Job drawing, mm, ordinate dimensions from the low corner. One solid piece. A direction names the side the tool comes from. Round coordinates to 2 decimals unless told otherwise and drop trailing zeros. Loops run counter-clockwise (first coordinate to the right, second up) from the corner with the lowest first, then second, coordinate; pieces in that order, holes last. Notation, with made-up numbers: M -8.75,57.5 L 6.25,57.5 A19 ccw 6.25,61.5 Z; hole C 40.25,71 d8. An arc over 180 degrees is marked long. One line per item, written item: value.
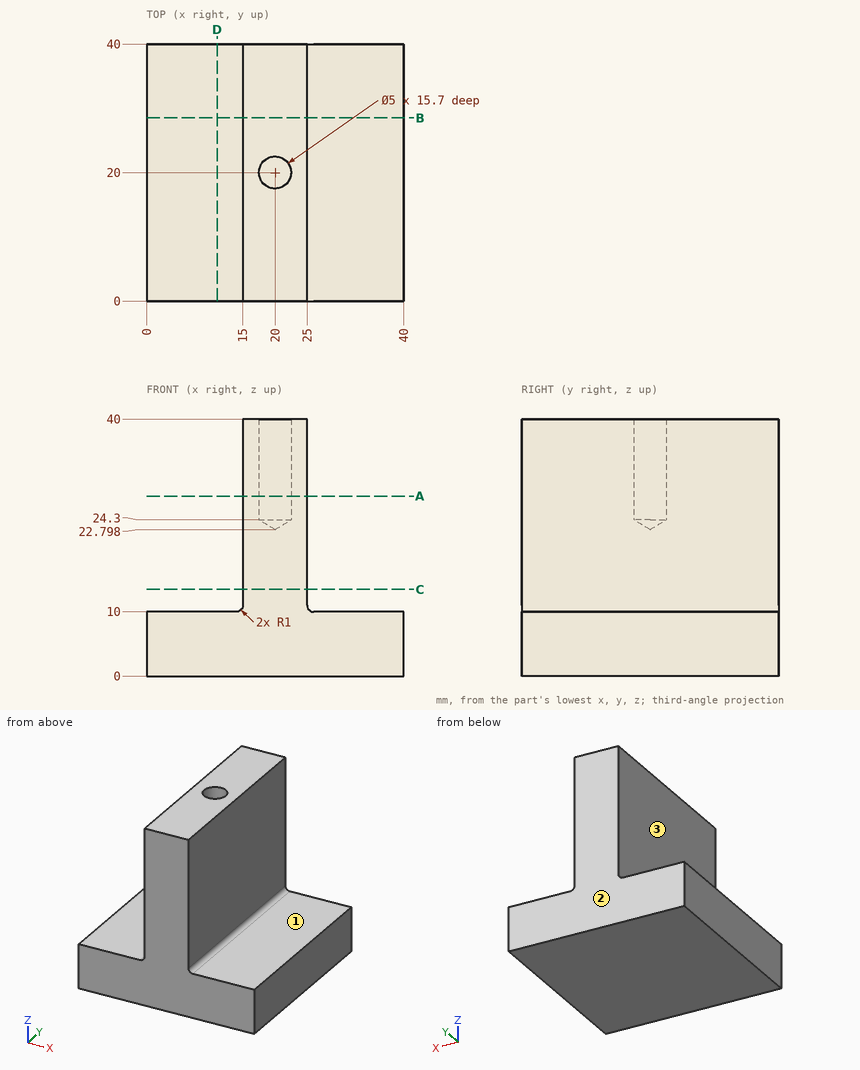
Item 1: Drop flat-ended pins along their axis: P1, Ø7, axis at x = 10, y = 11, coming from the +Z side; P2, Ø1.5, axis at y = 34, z = 12.5, coming from the +X side; P3, Ø14.5, axis at y = 25.5, z = 24, coming from the -X side. Give the stop position or say it passes through.
Check values:
P1: stops at z = 10
P2: stops at x = 25
P3: stops at x = 15
Item 2: Slice it at B-B, the plane y = 28.5. Give the cut face in (x, z).
Check values:
outline: M 0,0 L 40,0 L 40,10 L 26,10 A1 cw 25,11 L 25,40 L 15,40 L 15,11 A1 cw 14,10 L 0,10 Z
Item 3: Which spindle directions (+Z, -Z, +X, -X, +Y, -Y) get a long thin tool onto all of the face, cutting with end or side? Do the marked faces 1, 2 and 3. Say none if no direction does.
Check values:
face 1: +Z, +X, +Y, -Y
face 2: +Z, -Z, +X, -X, +Y
face 3: +Z, -X, +Y, -Y
Item 4: Slice it at C-C, the plane z = 13.5. Give the cut face in (x, y).
Check values:
outline: M 15,0 L 25,0 L 25,40 L 15,40 Z
Item 5: Wall check: line 1 along Y through (x, z) = (20, 34.5); line 2 along X through (y, z) = (20, 31); line 3 along X through (y, z) = (35, 20). Give the ranges that are in metal, low to high.
Check values:
line 1: y = 0 to 17.5, 22.5 to 40
line 2: x = 15 to 17.5, 22.5 to 25
line 3: x = 15 to 25
Item 6: Slice it at A-A, the plane z = 28. Give the cut face in (x, y).
Check values:
outline: M 15,0 L 25,0 L 25,40 L 15,40 Z; hole C 20,20 d5
Item 7: Slice it at D-D, the plane x = 11. Give the cut face in (y, z).
Check values:
outline: M 0,0 L 40,0 L 40,10 L 0,10 Z
